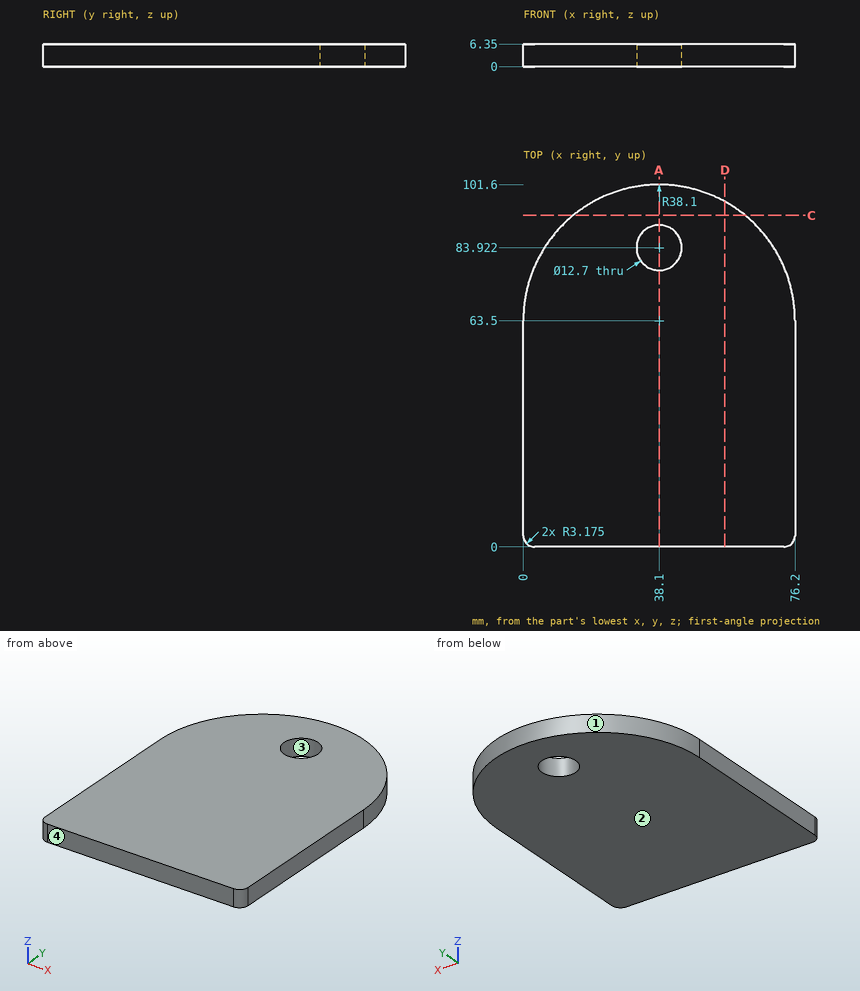
Job drawing, mm, ordinate dimensions from the low corner. One solid piece. Give positions to 0.01 mm unless a question says otherwise; leave off trailing zeros. Loops run counter-clockwise (first coordinate to the right, second up) from the corner with the lowest first, then second, coordinate; pieces in that order, holes last. Notation, with made-up numbers: M 20.5,82.25 L 28.5,82.25 A17 ccw 28.5,87.25 Z; hole C -22.75,-27 d1. An arc over 180 degrees is marked long. Answer in a Markdown table with one row per item. Add a question column.
Item 1: Mould opens along Y. For the marked faces 1, 2, 3 and 4 say: +Y half, -Y half, draft (parallel to the pull), parting line (faces both ways), or undercut.
Item 2: Band-saw the part on C-C on y = 93. Give the cut face in (x, z).
Item 3: Probe probe 1 along Y at (x, z) = (38.1, 1.5); probe 2 along Y at (x, z) = (60.5, 1.25); probe 3 along Y at (x, z) = (64.5, 2). List the from-to ranges inside material, lowest first.
Item 4: Band-saw the part on A-A on x = 38.1. Give the cut face in (y, z).
Item 5: Band-saw the part on D-D on x = 56.5. Give the cut face in (y, z), then the cut area to 3 significant figures.
Item 6: Drop flat-ended pins along their axis: P1, Ø3, axis at x = 35.5, z = 5.5, coming from the +Y side; P2, Ø2, axis at y = 86, z = 1, coming from the +X side (1 decimal). Give the stop position or say it passes through.
Reply:
| question | item | result |
|---|---|---|
| 1 | face 1 | +Y half |
| 1 | face 2 | draft |
| 1 | face 3 | undercut |
| 1 | face 4 | -Y half |
| 2 | outline | M 13.99,0 L 62.21,0 L 62.21,6.35 L 13.99,6.35 Z |
| 3 | probe 1 | y = 0 to 77.57, 90.27 to 101.6 |
| 3 | probe 2 | y = 0 to 94.32 |
| 3 | probe 3 | y = 0 to 90.97 |
| 4 | outline | M 0,0 L 77.57,0 L 77.57,6.35 L 0,6.35 Z; M 90.27,0 L 101.6,0 L 101.6,6.35 L 90.27,6.35 Z |
| 5 | outline | M 0,0 L 96.86,0 L 96.86,6.35 L 0,6.35 Z |
| 5 | area | 615 mm^2 |
| 6 | P1 | stops at y = 101.58 |
| 6 | P2 | stops at x = 69.6 |
